Check sheet for the modelled part. Datum: model origin and axes. Units: mm. A direction names the side the tool comes from. Round coordinates to 2 decimals unless told otherwise and drop trailing zeros. Write each loop counter-clockwise with the first axis right and the second up, starting at its lowest first coordinate (ties: lowest second). Pieces come first, ordered by that corner, then holes. Notation, with made-up numbers: (43, 6) -> (62, 6) arc R11 cw to (62, 27) -> close; hole circle Ø5 at (46, 23). An arc over 180 degrees is marked (long way). One line per item, written item: value.
from build123d import *

# Parameters (mm, degrees)
BOSS_EXTRUDE1_DEPTH       = 12.7
F_2_56_TAPPED_HOLE1_D     = 1.778
F_2_56_TAPPED_HOLE1_DEPTH = 3.175
F_2_56_TAPPED_HOLE1_TIP   = 0.53416509
CUT_EXTRUDE1_DEPTH        = 128.791284914
CUT_EXTRUDE2_DEPTH        = 3.81
F_2_56_TAPPED_HOLE2_D     = 1.778
F_8_CLEARANCE_HOLE1_D     = 4.4958
F_1_4_CLEARANCE_HOLE1_D   = 6.7564
LPATTERN1_COUNT           = 3
LPATTERN1_PITCH           = 25.4
SKETCH11_R                = 2.38125
CUT_EXTRUDE3_DEPTH        = 2.54


with BuildPart() as part:
    # Sketch1 → Boss-Extrude1 (new body)
    with BuildSketch(Plane.XY):
        with BuildLine():
            Line((0, 0), (127, 0))
            Line((127, 0), (127, 6.35))
            Line((127, 6.35), (0, 6.35))
            ThreePointArc((0, 6.35), (-3.175, 3.175), (0, 0))
        make_face()
    extrude(amount=BOSS_EXTRUDE1_DEPTH)

    # #2-56 Tapped Hole1
    with Locations(Plane(origin=(0, 3.175, 12.7), x_dir=(1, 0, 0), z_dir=(0, 0, 1))):
        with Locations((0, 0)):
            Hole(F_2_56_TAPPED_HOLE1_D / 2, depth=F_2_56_TAPPED_HOLE1_DEPTH)
            with Locations((0, 0, -(F_2_56_TAPPED_HOLE1_DEPTH + F_2_56_TAPPED_HOLE1_TIP / 2))):  # 118° drill point
                Cone(0, F_2_56_TAPPED_HOLE1_D / 2, F_2_56_TAPPED_HOLE1_TIP, mode=Mode.SUBTRACT)

    # Sketch6 → Cut-Extrude1 (cut, through all)
    with BuildSketch(Plane(origin=(0, 6.35, 0), x_dir=(1, 0, 0), z_dir=(0, 1, 0))):
        with BuildLine():
            Line((19.05, -4.445), (31.75, -4.445))
            ThreePointArc((31.75, -4.445), (33.655, -6.35), (31.75, -8.255))
            Line((31.75, -8.255), (19.05, -8.255))
            ThreePointArc((19.05, -8.255), (17.145, -6.35), (19.05, -4.445))
        make_face()
    extrude(amount=-CUT_EXTRUDE1_DEPTH, mode=Mode.SUBTRACT)

    # Sketch7 → Cut-Extrude2 (cut)
    with BuildSketch(Plane(origin=(0, 6.35, 0), x_dir=(1, 0, 0), z_dir=(0, 1, 0))):
        with BuildLine():
            Line((28.3845, -10.31875), (28.3845, -2.38125))
            ThreePointArc((28.3845, -2.38125), (29.21, -1.55575), (30.0355, -2.38125))
            Line((30.0355, -2.38125), (30.0355, -10.31875))
            ThreePointArc((30.0355, -10.31875), (29.21, -11.14425), (28.3845, -10.31875))
        make_face()
        with BuildLine():
            Line((25.8445, -10.31875), (25.8445, -2.38125))
            ThreePointArc((25.8445, -2.38125), (26.67, -1.55575), (27.4955, -2.38125))
            Line((27.4955, -2.38125), (27.4955, -10.31875))
            ThreePointArc((27.4955, -10.31875), (26.67, -11.14425), (25.8445, -10.31875))
        make_face()
    extrude(amount=-CUT_EXTRUDE2_DEPTH, mode=Mode.SUBTRACT)

    # #2-56 Tapped Hole2 (through all)
    with Locations(Plane(origin=(8.89, 6.35, 6.35), x_dir=(0, 0, 1), z_dir=(0, 1, 0))):
        with Locations((0, 0)):
            Hole(F_2_56_TAPPED_HOLE2_D / 2)

    # #8 Clearance Hole1 (through all)
    with Locations(Plane(origin=(120.65, 6.35, 6.35), x_dir=(0, 0, 1), z_dir=(0, 1, 0))):
        with Locations((0, 0)):
            f_8_clearance_hole1 = Hole(F_8_CLEARANCE_HOLE1_D / 2)

    # 1/4 Clearance Hole1 (through all)
    with Locations(Plane(origin=(107.95, 6.35, 6.35), x_dir=(0, 0, 1), z_dir=(0, 1, 0))):
        with Locations((0, 0)):
            f_1_4_clearance_hole1 = Hole(F_1_4_CLEARANCE_HOLE1_D / 2)

    # LPattern1: #8 Clearance Hole1, 1/4 Clearance Hole1 ×3
    with Locations(*[(-i * LPATTERN1_PITCH, 0, 0) for i in range(1, LPATTERN1_COUNT)]):
        add(f_8_clearance_hole1, mode=Mode.SUBTRACT)
        add(f_1_4_clearance_hole1, mode=Mode.SUBTRACT)

    # Sketch11 → Cut-Extrude3 (cut)
    with BuildSketch(Plane(origin=(0, 6.35, 0), x_dir=(1, 0, 0), z_dir=(0, 1, 0))):
        with Locations(Location((8.89, -6.35, 0), (0, 0, 270))):
            Circle(SKETCH11_R)
    extrude(amount=-CUT_EXTRUDE3_DEPTH, mode=Mode.SUBTRACT)


solid = part.part
Item 1: Sectioned sample at A-A on x = 82.55. Enter the section's corners in (y, z).
Answer:
outline: (0, 0) -> (6.35, 0) -> (6.35, 2.97) -> (0, 2.97) -> close; (0, 9.73) -> (6.35, 9.73) -> (6.35, 12.7) -> (0, 12.7) -> close
Item 2: Thickness scan on line 1 (Z direction, x = 19, y = 4.75); line 2 (X direction, y = 1, z = 3.75); line 3 (X direction, y = 3.75, z = 2.25) (1 decimal). Record the ranges inside material, lowest first.
Answer:
line 1: z = 0 to 4.45, 8.25 to 12.7
line 2: x = -2.31 to 54.99, 59.31 to 80.39, 84.71 to 105.79, 110.11 to 127
line 3: x = -3.1 to 25.9, 27.5 to 28.4, 30 to 127
Item 3: Depth check by flat-ended pin: P1, Ø1.8, axis at x = 27, z = 9.5, coming from the +Y side; P2, Ø1.4, axis at x = 9, z = 7.5, coming from the +Y side; P3, Ø0.8, axis at x = 27, z = 2.5, coming from the +Y side. Enter the tip coordinate at first touch or a pass-through.
Answer:
P1: stops at y = 6.35
P2: stops at y = 3.81
P3: stops at y = 2.54
Item 4: Tool access check on faces 1 (the flat face through (25.844, 4, 3)), 2 (the flat face through (25, 3, 8.255)), 3 (the flat face through (64, 6.35, 6)). Record the directions out of +Z, -Z, +X, -X, +Y, -Y that give a thin tool (end or side, any length) a straight path to the whole face; none if there is none.
Answer:
face 1: +Y
face 2: +Y, -Y
face 3: +Z, -Z, +X, -X, +Y
Item 5: Mould release check, pull along Z, two halves, no side actions. Record for faces 4 (the flat face through (61, 3, 12.7)), 5 (the flat face through (8.9, 3.81, 7.4)), 6 (the flat face through (127, 3, 6)), 7 (the flat face through (61, 3, 0)): pulls with the +Z half, pulls with the -Z half, needs draft (parallel to the pull), parting line crosses it, or undercut.
Answer:
face 4: pulls with the +Z half
face 5: undercut
face 6: needs draft
face 7: pulls with the -Z half
Item 6: Sectioned sample at B-B on y = 1. Count the separate pieces of the cut face and the enclosed holes in it, and give its area (3 significant figures).
Answer:
separate pieces: 1
enclosed holes: 8
area: 1,420 mm^2
Item 7: Sectioned sample at C-C on x = 59. Enter the section's corners in (y, z), and give its area (3 significant figures).
Answer:
outline: (0, 0) -> (6.35, 0) -> (6.35, 3.52) -> (0, 3.52) -> close; (0, 9.18) -> (6.35, 9.18) -> (6.35, 12.7) -> (0, 12.7) -> close
area: 44.7 mm^2
